For this review, take the finished solid that the model builds, in its own axes (mm). Face numbers are marked on the shaded views. A direction names the side the tool comes from. Coordinates: 2 decimals unless noted, no trailing zeros. Loops run counter-clockwise (first coordinate to the right, second up) from the corner with the lowest first, then second, coordinate; pieces in that order, holes last. Notation, with made-up numbers: M 2.25,47 L 16.25,47 A9 cw 16.25,57 Z; hole C 9.25,15.5 d4. An arc over 180 degrees is marked long. Write each question's results on one line, items separated by ' | '. Start each with the question number.
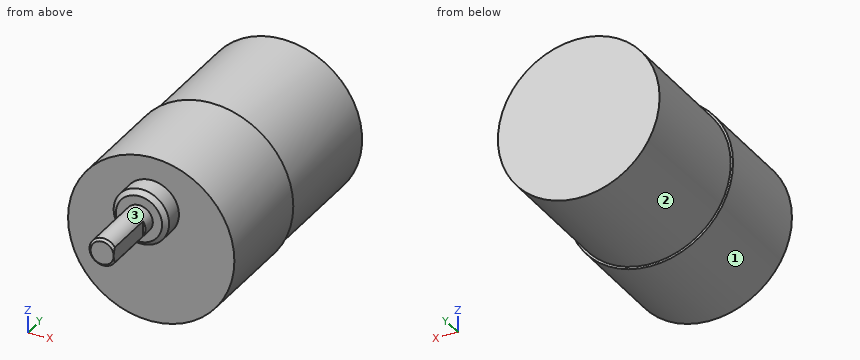
```python
from build123d import *

# Parameters (mm, degrees)
F0_R      = 18
F1_DEPTH  = 24
F2_R      = 6
F3_DEPTH  = 5
F4_SIZE   = 1
F5_R      = 3
F6_DEPTH  = 15
F7_SIZE   = 0.5
F8_W      = 1.9986620047
F8_H      = 4.7967880898
F9_DEPTH  = 12
F10_R     = 17.5
F11_DEPTH = 29


with BuildPart() as f1:
    # F0 (on Front) → F1 (new body)
    with BuildSketch(Plane.XZ):
        Circle(F0_R)
    extrude(amount=F1_DEPTH)

    # F2 (on face) → F3 (join)
    with BuildSketch(Plane.XZ.offset(24)):
        with Locations((0, 7)):
            Circle(F2_R)
    extrude(amount=F3_DEPTH)

    # F4
    f4_edges = [f1.edges().sort_by_distance(p)[0] for p in [
        (-6, -29, 7),
    ]]
    chamfer(f4_edges, length=F4_SIZE)

    # F5 (on face) → F6 (join)
    with BuildSketch(Plane.XZ.offset(29)):
        with Locations((0, 7)):
            Circle(F5_R)
    extrude(amount=F6_DEPTH)

    # F7
    f7_edges = [f1.edges().sort_by_distance(p)[0] for p in [
        (-3, -44, 7),
    ]]
    chamfer(f7_edges, length=F7_SIZE)

    # F8 (on face) → F9 (cut)
    with BuildSketch(Plane.XZ.offset(44)):
        with Locations((3.4993309465, 6.97000045)):
            Rectangle(F8_W, F8_H)
    extrude(amount=-F9_DEPTH, mode=Mode.SUBTRACT)

    # F10 (on face) → F11 (join)
    with BuildSketch(Plane(origin=(0, 0, 0), x_dir=(-1, 0, 0), z_dir=(0, 1, 0))):
        Circle(F10_R)
    extrude(amount=F11_DEPTH)


solid = f1.part
```
Q1. For the marked faces 1, 2 and 3, list the 3-axis set-ups (+Z, -Z, +X, -X, +Y, -Y) from which the entire face can be reached by the end or side of a thin tool; tool diameter is ignored.
Q2. Take a section at B-B, the plane y = -8.5. Give the boundary of the cut face in (x, z).
Q3. Insertion check: P1, Ø1.5, axis at y = -35.5, z = 6, coming from the -X side; P2, Ø10, axis at y = 17.5, z = -0.5, coming from the +X side; P3, Ø1.5, axis at x = -12.5, y = -26.5, coming from the +Z side; P4, Ø3.5, axis at y = -40.5, z = 7.5, coming from the +X side. Each pin has a flat end and moves straight along its axis. Give the tip position at first contact, or say it passes through.
Q4. Take a section at A-A, the plane x = 0. Give the boundary of the cut face in (y, z), then the cut area to 3 significant figures.
Q5. To check wall thickness, follow line 1 along Y through (x, z) = (-5.5, 14.5); line 2 along Y through (x, z) = (-4.5, 8); line 3 along Z through (x, y) = (9.5, 7). State the ranges of each line that lie inside material, in increasing order.
Q6. Take a section at C-C, the plane z = -12. Give the boundary of the cut face in (x, y), then the cut area to 3 significant figures.
Q7. Take a section at D-D, the plane x = -12.5. Give the boundary of the cut face in (y, z).
Results:
1) face 1: +Y, -Y | face 2: +Y | face 3: -Y
2) outline: C 0,0 d36
3) P1: x = -2.99 | P2: x = 17.5 | P3: through | P4: x = 2.5
4) outline: M -44,4.5 L -43.5,4 L -29,4 L -29,2 L -28,1 L -24,1 L -24,-18 L 0,-18 L 0,-17.5 L 29,-17.5 L 29,17.5 L 0,17.5 L 0,18 L -24,18 L -24,13 L -28,13 L -29,12 L -29,10 L -43.5,10 L -44,9.5 Z | area: 2,030 mm^2
5) line 1: -24 to 29 | line 2: -29 to 29 | line 3: -14.7 to 14.7
6) outline: M -13.42,-24 L 13.42,-24 L 13.42,0 L 12.74,0 L 12.74,29 L -12.74,29 L -12.74,0 L -13.42,0 Z | area: 1,380 mm^2
7) outline: M -24,-12.95 L 0,-12.95 L 0,-12.25 L 29,-12.25 L 29,12.25 L 0,12.25 L 0,12.95 L -24,12.95 Z
